```python
from build123d import *

# Parameters (mm, degrees)
F3_R     = 0.889
F4_DEPTH = 6.35


with BuildPart() as f1:
    # F0 (on Right) → F1 (revolve)
    with BuildSketch(Plane.YZ):
        Polygon((-17.4625, 2.54), (-3.175, 2.54), (-3.175, 5.334), (0, 5.334), (0, 6.985), (-17.4625, 6.985), align=None)
    revolve(axis=Axis((0, 0, 6.1595), (0, 0, -1)))

    # F3 (on offset) → F4 (cut)
    with BuildSketch(Plane.YZ.offset(17.4625)):
        with Locations((0, 4.7625)):
            Circle(F3_R)
    extrude(amount=-F4_DEPTH, mode=Mode.SUBTRACT)


solid = f1.part
```
Can you work these out from the model? Positions are in its coordinate system, mm. A direction names the side the tool comes from. Coordinates: 2 decimals unless noted, no trailing zeros. Write each loop counter-clockwise with the first axis right and the second up, starting at its lowest first coordinate (ties: lowest second). Pieces come first, ordered by that corner, then holes. Notation, with made-up numbers: (38.25, 36) - (64.25, 36) arc R37 ccw to (64.25, 72) - close; hole circle Ø6 at (56, 13.5). An arc over 180 degrees is marked (long way). Return JSON: item names as keys, results as strings.
Q1. If we section it at C-C (z = 6.2): Please give me the cut outline in (x, y) (1 decimal).
Computed values:
{"outline": "circle Ø34.9 at (0, 0)"}
Q2. Thinking about a two-plate mould opening in Z: for faces 4 (the cylindrical face through (14.33, 0.48, 5.51)), 5 (the flat face through (0, -4, 2.54)), 6 (the flat face through (0, 0, 6.985)), which applies, +Z half, -Z half, draft (parallel to the pull), parting line (faces both ways), or undercut?
Computed values:
{"face 4": "undercut", "face 5": "-Z half", "face 6": "+Z half"}
Q3. On a 3-axis mill with a long thin cutter (end or side, diameter ignored), from which of +Z, -Z, +X, -X, +Y, -Y can I reach the whole of each face in a straight line? I mean faces 1 (the cylindrical face through (10.626, 13.858, 4.731)), 2 (the flat face through (11.112, 0, 5)), 3 (the flat face through (0, 0, 5.334)). Say none if no direction works.
Computed values:
{"face 1": "+Z, -Z", "face 2": "+X", "face 3": "-Z"}
Q4. Please list where these lines run through material, in increasing order: L1, parallel to X at y = 0, z = 4.45 (1 decimal); L2, parallel to Y at x = 0, z = 3.85 (1 decimal); L3, parallel to Z at x = 15, y = 0 (1 decimal). Write a range as from..to.
Computed values:
{"L1": "x = -17.5..-3.2, 3.2..11.1", "L2": "y = -17.5..-3.2, 3.2..17.5", "L3": "z = 2.5..3.9, 5.7..7"}
Q5. If we section it at B-B (y = 0): Please give me the cut outline in (x, z) (1 decimal).
Computed values:
{"outline": "(-17.5, 2.5) - (-3.2, 2.5) - (-3.2, 5.3) - (3.2, 5.3) - (3.2, 2.5) - (17.5, 2.5) - (17.5, 3.9) - (11.1, 3.9) - (11.1, 5.7) - (17.5, 5.7) - (17.5, 7) - (-17.5, 7) - close"}
Q6. I'm going to push flat-ended pins straight in: pin 1 Ø7 at (x, y) = (1.5, 0.5) entering from -Z; pin 2 Ø4 at (x, y) = (0, 0) entering from -Z. Where does each tip first touch, or does it pass through?
Computed values:
{"pin 1": "stops at z = 2.54", "pin 2": "stops at z = 5.33"}
Q7. If we section it at A-A (x = 0): Please give me the cut outline in (y, z) (1 decimal).
Computed values:
{"outline": "(-17.5, 2.5) - (-3.2, 2.5) - (-3.2, 5.3) - (3.2, 5.3) - (3.2, 2.5) - (17.5, 2.5) - (17.5, 7) - (-17.5, 7) - close"}
Q8. If we section it at D-D (x = -8): Please give me the cut outline in (y, z) (3 decimals), then the cut area to 3 significant figures.
Computed values:
{"outline": "(-15.522, 2.54) - (15.522, 2.54) - (15.522, 6.985) - (-15.522, 6.985) - close", "area": "138 mm2"}
